Check sheet for the drawn part. Datum: minimum x, y, z corner. Units: mm. Round coordinates to 2 decimals unless told otherwise and drop trailing zeros. Write each loop counter-clockwise with the first axis right and the second up, starting at its lowest first coordinate (ties: lowest second). Pieces come first, ordered by that corner, then holes. Notation, with made-up numbers: (-38, -34) - (8, -34) arc R24 cw to (8, -11) - close; hole circle Ø11 at (-22, -6.75). An arc over 180 degrees is marked (long way). Return JSON: item names as keys, results as strings. Group by question number.
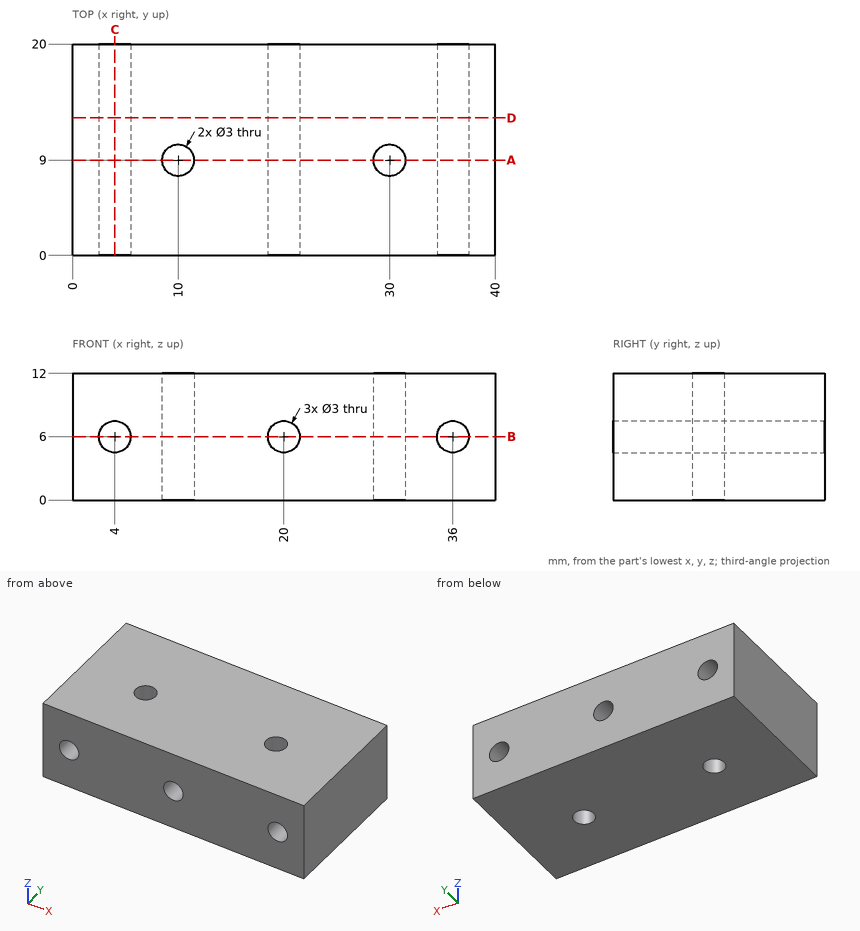
1. Section check D-D (y = 13). Enter the section's corners in (x, z).
2. Section check C-C (x = 4). Enter the section's corners in (y, z), and give its area (3 significant figures).
3. Material ranges on line 1 along X through (y, z) = (15, 6); line 2 along X through (y, z) = (14.5, 5.5); line 3 along Y through (x, z) = (10.5, 4.5), recorded low to high.
4. Section check B-B (z = 6). Enter the section's corners in (x, y), and give its area (3 significant figures).
5. Section check A-A (y = 9). Enter the section's corners in (x, z), and give its area (3 significant figures).
Result sheet:
{
 "1": {"outline": "(0, 0) - (40, 0) - (40, 12) - (0, 12) - close; hole circle Ø3 at (4, 6); hole circle Ø3 at (20, 6); hole circle Ø3 at (36, 6)"},
 "2": {"outline": "(0, 0) - (20, 0) - (20, 4.5) - (0, 4.5) - close; (0, 7.5) - (20, 7.5) - (20, 12) - (0, 12) - close", "area": "180 mm²"},
 "3": {"line 1": "x = 0 to 2.5, 5.5 to 18.5, 21.5 to 34.5, 37.5 to 40", "line 2": "x = 0 to 2.59, 5.41 to 18.59, 21.41 to 34.59, 37.41 to 40", "line 3": "y = 0 to 7.59, 10.41 to 20"},
 "4": {"outline": "(0, 0) - (2.5, 0) - (2.5, 20) - (0, 20) - close; (5.5, 0) - (18.5, 0) - (18.5, 20) - (5.5, 20) - close; (21.5, 0) - (34.5, 0) - (34.5, 20) - (21.5, 20) - close; (37.5, 0) - (40, 0) - (40, 20) - (37.5, 20) - close; hole circle Ø3 at (10, 9); hole circle Ø3 at (30, 9)", "area": "606 mm²"},
 "5": {"outline": "(0, 0) - (8.5, 0) - (8.5, 12) - (0, 12) - close; (11.5, 0) - (28.5, 0) - (28.5, 12) - (11.5, 12) - close; (31.5, 0) - (40, 0) - (40, 12) - (31.5, 12) - close; hole circle Ø3 at (4, 6); hole circle Ø3 at (20, 6); hole circle Ø3 at (36, 6)", "area": "387 mm²"}
}
